```python
from build123d import *

# Parameters (mm, degrees)
CUT_EXTRUDE1_DEPTH      = 11.43
SKETCH3_R               = 3.175
CUT_EXTRUDE2_DEPTH      = 51.497474194
CUT_EXTRUDE3_DEPTH      = 48.941448664
CUT_EXTRUDE3_DEPTH_BACK = 48.941448664
SKETCH4_W               = 5.08
SKETCH4_H               = 1.27
FILLET1_R               = 1.905


with BuildPart() as part:
    # Sketch1 → Revolve1 (revolve)
    with BuildSketch(Plane.XY, mode=Mode.PRIVATE) as revolve1_sk:
        with BuildLine():
            Line((0, 0), (0, 5.602635041))
            Line((0, 5.602635041), (-2.54, 5.602635041))
            Line((-2.54, 5.602635041), (-2.54, 36.83))
            Line((-2.54, 36.83), (0, 36.83))
            Line((0, 36.83), (0, 44.45))
            ThreePointArc((0, 44.45), (-8.980256121, 40.730256121), (-12.7, 31.75))
            Line((-12.7, 31.75), (-12.7, 0))
            Line((-12.7, 0), (0, 0))
        make_face()
    revolve(revolve1_sk.sketch.rotate(Axis((0, 0, 0), (0, 1, 0)), 270), axis=Axis((0, 0, 0), (0, 1, 0)))

    # Sketch2 → Cut-Extrude1 (cut)
    with BuildSketch(Plane.XZ):
        with BuildLine():
            Line((-2.54, 12.443407893), (-2.54, -12.443407893))
            ThreePointArc((-2.54, -12.443407893), (0, -12.7), (2.54, -12.443407893))
            Line((2.54, -12.443407893), (2.54, 12.443407893))
            ThreePointArc((2.54, 12.443407893), (0, 12.7), (-2.54, 12.443407893))
        make_face()
        with BuildLine():
            Line((-7.62, 10.16), (-7.62, -10.16))
            ThreePointArc((-7.62, -10.16), (-12.7, 0), (-7.62, 10.16))
        make_face()
        with BuildLine():
            Line((7.62, 10.16), (7.62, -10.16))
            ThreePointArc((7.62, -10.16), (12.7, 0), (7.62, 10.16))
        make_face()
    extrude(amount=-CUT_EXTRUDE1_DEPTH, mode=Mode.SUBTRACT)

    # Sketch3 → Cut-Extrude2 (cut, through all)
    with BuildSketch(Plane.ZY.offset(7.62)):
        with Locations((0, 5.08)):
            Circle(SKETCH3_R)
        with BuildLine():
            Line((0, 0), (12.443407893, 0))
            Line((12.443407893, 0), (12.443407893, 11.43))
            Line((12.443407893, 11.43), (3.796422114, 1.704562379))
            ThreePointArc((3.796422114, 1.704562379), (2.080766311, 0.445691901), (0, 0))
        make_face()
    extrude(amount=-CUT_EXTRUDE2_DEPTH, mode=Mode.SUBTRACT)

    # Sketch4 → Cut-Extrude3 (cut, two sides: drawn at the far end of the back side and taken through both)
    with BuildSketch(Plane.XY.offset(-CUT_EXTRUDE3_DEPTH_BACK)):
        with Locations((0, 31.115)):
            Rectangle(SKETCH4_W, SKETCH4_H)
        with Locations((0, 36.195)):
            Rectangle(SKETCH4_W, SKETCH4_H)
    extrude(amount=CUT_EXTRUDE3_DEPTH + CUT_EXTRUDE3_DEPTH_BACK, mode=Mode.SUBTRACT)

    # Fillet1
    # the kernel refuses this fillet: 1.905 mm, written as the material it takes off along each edge
    with BuildSketch(Plane(origin=(0, 31.75, 0), x_dir=(-0.6006287696946434, 0, 0.7995280364159214), z_dir=(-0.7995280364159214, 0, -0.6006287696946434))) as fillet1_piece_1_section:
        with BuildLine():
            CenterArc((10.625582337, 1.905), FILLET1_R, 270, 100.164248622)
            Line((10.625582337, 0), (12.7, 0))
            ThreePointArc((12.7, 0), (12.650073138, 1.125010933), (12.500685102, 2.241176471))
        make_face()
    fillet1_piece_1 = revolve(axis=Axis((0, 31.75, 0), (0, 1, 0)), revolution_arc=73.829886486, mode=Mode.PRIVATE)
    fillet1_piece_1 = split(fillet1_piece_1, bisect_by=Plane(origin=(-2.54, 32.266908465, 12.1243087), z_dir=(1, 0, 0)), keep=Keep.TOP, mode=Mode.PRIVATE)
    fillet1_piece_1 = split(fillet1_piece_1, bisect_by=Plane(origin=(2.54, 32.266908465, 12.1243087), z_dir=(-1, 0, 0)), keep=Keep.TOP, mode=Mode.PRIVATE)
    add(fillet1_piece_1, mode=Mode.SUBTRACT)
    with BuildSketch(Plane(origin=(0, 35.56, 0), x_dir=(0.5180820301307622, 0, 0.8553309359865267), z_dir=(0.8553309359865267, 0, -0.5180820301307622))) as fillet1_piece_2_section:
        with BuildLine():
            CenterArc((10.625582337, 1.905), FILLET1_R, 270, 79.835751378)
            Line((10.625582337, 0), (12.115027858, 0))
            ThreePointArc((12.115027858, 0), (12.332827452, 0.778273257), (12.500685102, 1.568823529))
        make_face()
    fillet1_piece_2 = revolve(axis=Axis((0, 35.56, 0), (0, -1, 0)), revolution_arc=62.407371172, mode=Mode.PRIVATE)
    fillet1_piece_2 = split(fillet1_piece_2, bisect_by=Plane(origin=(-2.54, 35.21222625, 11.799196002), z_dir=(1, 0, 0)), keep=Keep.TOP, mode=Mode.PRIVATE)
    fillet1_piece_2 = split(fillet1_piece_2, bisect_by=Plane(origin=(2.54, 35.21222625, 11.799196002), z_dir=(-1, 0, 0)), keep=Keep.TOP, mode=Mode.PRIVATE)
    add(fillet1_piece_2, mode=Mode.SUBTRACT)
    with BuildSketch(Plane(origin=(0, 35.56, 0), x_dir=(0, 0, -1), z_dir=(-1, 0, 0))) as fillet1_piece_3_section:
        with BuildLine():
            CenterArc((10.625582337, 1.905), FILLET1_R, 270, 79.835751378)
            Line((10.625582337, 0), (12.115027858, 0))
            ThreePointArc((12.115027858, 0), (12.332827452, 0.778273257), (12.500685102, 1.568823529))
        make_face()
    fillet1_piece_3 = revolve(axis=Axis((0, 35.56, 0), (0, -1, 0)), revolution_arc=31.203269463, mode=Mode.PRIVATE)
    fillet1_piece_3 = split(fillet1_piece_3, bisect_by=Plane(origin=(2.54, 35.212226268, -11.799195909), z_dir=(-1, 0, 0)), keep=Keep.TOP, mode=Mode.PRIVATE)
    add(fillet1_piece_3, mode=Mode.SUBTRACT)
    with BuildSketch(Plane(origin=(0, 31.75, 0), x_dir=(0, 0, -1), z_dir=(1, 0, 0))) as fillet1_piece_4_section:
        with BuildLine():
            CenterArc((10.625582337, 1.905), FILLET1_R, 270, 100.164248622)
            Line((10.625582337, 0), (12.7, 0))
            ThreePointArc((12.7, 0), (12.650073138, 1.125010933), (12.500685102, 2.241176471))
        make_face()
    fillet1_piece_4 = revolve(axis=Axis((0, 31.75, 0), (0, 1, 0)), revolution_arc=36.914440828, mode=Mode.PRIVATE)
    fillet1_piece_4 = split(fillet1_piece_4, bisect_by=Plane(origin=(-2.54, 32.26690841, -12.124308672), z_dir=(1, 0, 0)), keep=Keep.TOP, mode=Mode.PRIVATE)
    add(fillet1_piece_4, mode=Mode.SUBTRACT)
    with BuildSketch(Plane(origin=(0, 31.75, 0), x_dir=(0.6006217587640484, 0, -0.799533303183289), z_dir=(0.799533303183289, 0, 0.6006217587640484))) as fillet1_piece_5_section:
        with BuildLine():
            CenterArc((10.625582337, 1.905), FILLET1_R, 270, 100.164248622)
            Line((10.625582337, 0), (12.7, 0))
            ThreePointArc((12.7, 0), (12.650073138, 1.125010933), (12.500685102, 2.241176471))
        make_face()
    fillet1_piece_5 = revolve(axis=Axis((0, 31.75, 0), (0, 1, 0)), revolution_arc=36.914440828, mode=Mode.PRIVATE)
    fillet1_piece_5 = split(fillet1_piece_5, bisect_by=Plane(origin=(2.54, 32.266908503, -12.124308915), z_dir=(-1, 0, 0)), keep=Keep.TOP, mode=Mode.PRIVATE)
    add(fillet1_piece_5, mode=Mode.SUBTRACT)
    with BuildSketch(Plane(origin=(0, 35.56, 0), x_dir=(-0.5180758180945625, 0, -0.8553346986447177), z_dir=(-0.8553346986447177, 0, 0.5180758180945625))) as fillet1_piece_6_section:
        with BuildLine():
            CenterArc((10.625582337, 1.905), FILLET1_R, 270, 79.835751378)
            Line((10.625582337, 0), (12.115027858, 0))
            ThreePointArc((12.115027858, 0), (12.332827452, 0.778273257), (12.500685102, 1.568823529))
        make_face()
    fillet1_piece_6 = revolve(axis=Axis((0, 35.56, 0), (0, -1, 0)), revolution_arc=31.203269463, mode=Mode.PRIVATE)
    fillet1_piece_6 = split(fillet1_piece_6, bisect_by=Plane(origin=(-2.54, 35.212226169, -11.799196271), z_dir=(1, 0, 0)), keep=Keep.TOP, mode=Mode.PRIVATE)
    add(fillet1_piece_6, mode=Mode.SUBTRACT)


solid = part.part
```
Check sheet for the modelled part. Datum: model origin and axes. Units: mm. A direction names the side the tool comes from. Round coordinates to 2 decimals unless told otherwise and drop trailing zeros. Loops run counter-clockwise (first coordinate to the right, second up) from the corner with the lowest first, then second, coordinate; pieces in that order, holes last. Notation, with made-up numbers: M 16.5,88 L 72.5,88 A33 ccw 72.5,118 Z; hole C 41.5,16 d2. An arc over 180 degrees is marked long. Answer as a JSON object with one key per item and string values.
1. Section check C-C (z = -6). Record the boundary of the cut face in (x, y).
Reply:
{"outline": "M -11.19,11.43 L -7.62,11.43 L -7.62,0 L -2.54,0 L -2.54,11.43 L 2.54,11.43 L 2.54,0 L 7.62,0 L 7.62,11.43 L 11.19,11.43 L 11.19,31.75 A11.19 ccw -11.19,31.75 Z; hole M -2.54,30.48 L 2.54,30.48 L 2.54,31.75 L -2.54,31.75 Z; hole M -2.54,35.56 L 2.54,35.56 L 2.54,36.83 L -2.54,36.83 Z"}
2. Access from +Z, -Z, +X, -X, +Y, -Y to the whole of each face (thin tool, end or side, straight path). Record for faces 5 (the flat face through (0, 31.75, 6)), 6 (the flat face through (-2.54, 8, -3)), 7 (the flat face through (7.62, 8, -2)), 8 (the cylindrical face through (-2.52, 33.68, 0.33)).
Reply:
{"face 5": "+Z, -Z", "face 6": "+Z, -Z, -Y", "face 7": "+Z, -Z, +X, -Y", "face 8": "-Y"}
3. Mould release check, pull along X, two halves, no side actions. Record for faces 1 (the flat face through (-10, 11.43, 0)), 2 (the flat face through (-7.62, 8, -2)), 3 (the flat face through (0, 30.48, 8)), 4 (the flat face through (0, 35.56, -7)): pulls with the +X half, pulls with the -X half, needs draft (parallel to the pull), parting line crosses it, or undercut.
Reply:
{"face 1": "needs draft", "face 2": "pulls with the -X half", "face 3": "undercut", "face 4": "undercut"}
4. Gauge pin test, flat ends, axial feed: P1, Ø1, axis at x = -5.5, y = 11.5, coming from the -Z side; P2, Ø5.5, axis at x = -0.5, z = 3.5, coming from the -Y side; P3, Ø0.5, axis at y = 35, z = 11, coming from the +X side. Record the tip position at first contact, or that the pin passes through.
Reply:
{"P1": "stops at z = -11.67", "P2": "stops at y = 0.28", "P3": "stops at x = 5.95"}
5. Scan lines: line 1 (Y direction, x = -2.5, z = 7.5); line 2 (Y direction, x = 0.5, z = -3.25); line 3 (X direction, y = 9.5, z = -6.5). Record each from-to range of solid material in increasing order.
Reply:
{"line 1": "y = 11.43 to 30.48, 31.75 to 35.56, 36.83 to 41.69", "line 2": "y = 11.43 to 30.48, 31.75 to 35.56, 36.83 to 44.02", "line 3": "x = -7.62 to -2.54, 2.54 to 7.62"}
6. Section check B-B (x = -3). Record the boundary of the cut face in (y, z) (3 decimals), plus the area to 3 significant figures.
Reply:
{"outline": "M 0,-12.341 L 31.75,-12.341 A12.341 ccw 31.75,12.341 L 11.314,12.341 L 1.705,3.796 A5.08 ccw 0,0 Z; hole C 5.08,0 d6.35", "area": "934 mm²"}
7. Section check A-A (y = 6). Record the boundary of the cut face in (x, z).
Reply:
{"outline": "M -7.62,-10.16 A12.7 ccw -2.54,-12.44 L -2.54,-3.04 L -7.62,-3.04 Z; M -7.62,3.04 L -2.54,3.04 L -2.54,7.62 L -7.62,7.62 Z; M 2.54,-12.44 A12.7 ccw 7.62,-10.16 L 7.62,-3.04 L 2.54,-3.04 Z; M 2.54,3.04 L 7.62,3.04 L 7.62,7.62 L 2.54,7.62 Z"}
8. Section check D-D (y = 12). Record the boundary of the cut face in (x, z).
Reply:
{"outline": "C 0,0 d25.4; hole C 0,0 d5.08"}
